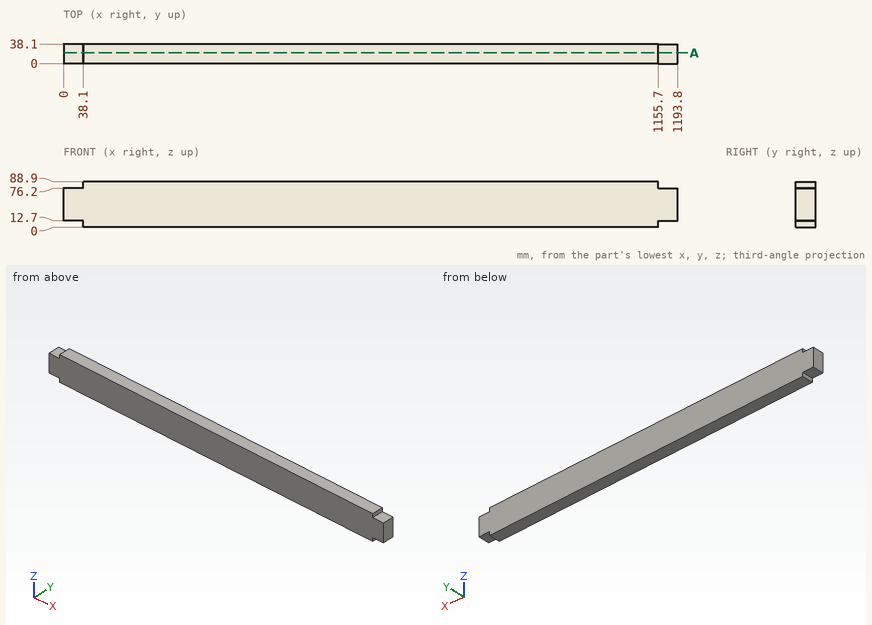
Could you check a few things on this drawing? It's one solid part, dimensions in mm from its lowest x, y, z. Give positions to 0.01 mm unless a question says otherwise; leave off trailing zeros. Write each loop counter-clockwise with the first axis right and the second up, starting at its lowest first coordinate (ties: lowest second). Pieces come first, ordered by that corner, then holes. Notation, with made-up numbers: (18.5, 8) -> (76.5, 8) arc R15 cw to (76.5, 26) -> close; hole circle Ø7 at (85.5, -14). An arc over 180 degrees is marked (long way). Answer as CSV lines item,"result". Start each with the question number.
(1) Please list where this line runs through material, in increasing order: line 1 (X direction, y = 21.5, z = 79).
(2) If we section it at A-A, the plane y = 21: Write out the boundary of the cut face in (x, z).
(3) I'm going to push flat-ended pins straight in: pin 1 Ø12 at (y, z) = (23, 57) entering from -X; pin 2 Ø10 at (y, z) = (21, 7) entering from +X; pin 3 Ø19 at (x, y) = (1176, 17.5) entering from -Z; pin 4 Ø6.5 at (y, z) = (27, 4) entering from -X. Where does each tip first touch, or does it pass through?
Answer list:
1,line 1,"38.1 to 1155.7"
2,outline,"(0, 12.7) -> (38.1, 12.7) -> (38.1, 0) -> (1155.7, 0) -> (1155.7, 12.7) -> (1193.8, 12.7) -> (1193.8, 76.2) -> (1155.7, 76.2) -> (1155.7, 88.9) -> (38.1, 88.9) -> (38.1, 76.2) -> (0, 76.2) -> close"
3,pin 1,"x = 0"
3,pin 2,"x = 1155.7"
3,pin 3,"z = 12.7"
3,pin 4,"x = 38.1"
